Input: dimensioned drawing with shaded views. Units: mm. Origin: part minimum x, y, z. A direction names the side the tool comes from. Round coordinates to 2 decimals unless told otherwise and drop trailing zeros. Write each loop counter-clockwise with the first axis right and the second up, starting at its lowest first coordinate (ties: lowest second). Pieces come first, ordered by that corner, then holes. Notation, with made-up numbers: (-20.5, 6) - (34.5, 6) arc R14 cw to (34.5, 10) - close; hole circle Ø3 at (37.25, 33). An arc over 180 degrees is marked (long way). Use one line per item in the form item = value.
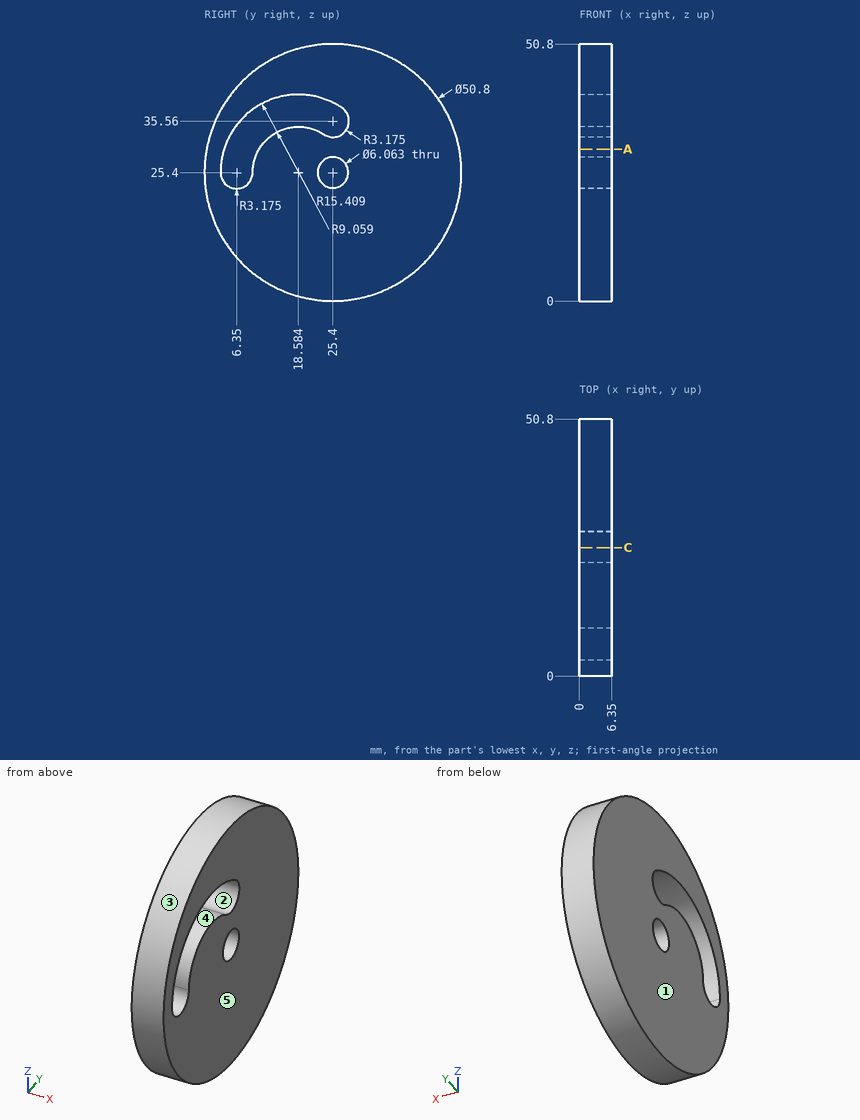
(1) Material intervals for L1, parallel to Y at x = 5.25, z = 25.4 (1 decimal); L2, parallel to Z at x = 5.5, y = 14 (1 decimal); L3, parallel to Z at x = 3, y = 13 (1 decimal), sorted ascending.
Derived:
L1 = 0 to 3.2, 9.5 to 22.4, 28.4 to 50.8
L2 = 2.7 to 33.2, 40.1 to 48.1
L3 = 3.2 to 32.5, 39.8 to 47.6
(2) Cut plane C-C on y = 25.4. Count the separate pieces of the cut face and the enclosed holes in it, then the cut area to 3 significant figures.
Derived:
separate_pieces = 3
enclosed_holes = 0
area = 241 mm^2
(3) Cut plane A-A on z = 30. Output: boundary loops of the cut face in (x, y).
Derived:
outline = (0, 0.42) - (6.35, 0.42) - (6.35, 3.88) - (0, 3.88) - close; (0, 10.78) - (6.35, 10.78) - (6.35, 50.38) - (0, 50.38) - close
(4) First-contact query: pin 1 Ø2 at (x, z) = (4.5, 41) entering from -Y (1 decimal); pin 2 Ø3.5 at (y, z) = (25.4, 25.4) entering from -X (3 decimals). Flat tips, straight axial feed; report the tip coordinate or a pass-through.
Derived:
pin_1 = 4.6
pin_2 = through
(5) Draft query along Y for the marked faces 1, 2 and 3. Return one class per face: released by +Y, released by -Y, zero draft, split by the parting line, or undercut.
Derived:
face_1 = zero draft
face_2 = undercut
face_3 = split by the parting line
(6) Access query for the marked faces 4 and 5. Directions: +Z, -Z, +X, -X, +Y, -Y. A direction counts if a zero-diameter tool reaches every point of the face in a straight line with its end or side. Return the directions, or none.
Derived:
face_4 = +X, -X
face_5 = +Z, -Z, +X, +Y, -Y
